Autodesk Inventor part; units mm, degrees
ref_plane "作業平面1" through (0, 0, 0) normal (0, 1, 0) x (-1, 0, 0)
ref_plane "YZ Plane" through (0, 0, 0) normal (1, 0, 0) x (0, 1, 0)
ref_plane "XY Plane" through (0, 0, 0) normal (0, 0, 1) x (1, 0, 0)
sketch "スケッチ1" plane through (0, 0, 0) normal (0, 0, 1) x (1, 0, 0)
  circle A0 centre (0, 0) radius 40
  circle A1 centre (0, 0) radius 2.5
  dimension "d0" = 80
  dimension "d1" = 5
extrude "押し出し1" add sketch "スケッチ1" along normal blind 3
sketch "スケッチ2" plane through (0, 0, 3) normal (0, 0, 1) x (1, 0, 0)
  circle A0 centre (0, 0) radius 8
  circle A1 centre (0, 0) radius 2.5
  circle A2 centre (0, 0) radius 35
  line L0 (3, 34.8712) -> (3, 7.4162)
  line L1 (-3, 7.4162) -> (-3, 34.8712)
  line L2 (-7.3654, 3.1227) -> (-26.779, 22.5363)
  line L3 (-22.5363, 26.779) -> (-3.1227, 7.3654)
  circle A3 centre (0, 0) radius 35
  circle A4 centre (0, 0) radius 8
  line L4 (-7.4162, -3) -> (-34.8712, -3)
  line L5 (-34.8712, 3) -> (-7.4162, 3)
  circle A5 centre (0, 0) radius 35
  circle A6 centre (0, 0) radius 8
  line L6 (-3.1227, -7.3654) -> (-22.5363, -26.779)
  line L7 (-26.779, -22.5363) -> (-7.3654, -3.1227)
  circle A7 centre (0, 0) radius 35
  circle A8 centre (0, 0) radius 8
  line L8 (3, -7.4162) -> (3, -34.8712)
  line L9 (-3, -34.8712) -> (-3, -7.4162)
  circle A9 centre (0, 0) radius 35
  circle A10 centre (0, 0) radius 8
  line L10 (7.3654, -3.1227) -> (26.779, -22.5363)
  line L11 (22.5363, -26.779) -> (3.1227, -7.3654)
  circle A11 centre (0, 0) radius 35
  circle A12 centre (0, 0) radius 8
  line L12 (7.4162, 3) -> (34.8712, 3)
  line L13 (34.8712, -3) -> (7.4162, -3)
  circle A13 centre (0, 0) radius 35
  circle A14 centre (0, 0) radius 8
  line L14 (3.1227, 7.3654) -> (22.5363, 26.779)
  line L15 (26.779, 22.5363) -> (7.3654, 3.1227)
  circle A15 centre (0, 0) radius 35
  circle A16 centre (0, 0) radius 8
  dimension "d4" = 16
  dimension "d5" = 70
  dimension "d6" = 3
  dimension "d7" = 6
  dimension "d10" = 360
extrude "押し出し2" cut sketch "スケッチ2" against normal blind 5 contours A0 L15 A2 L12 | L13 A2 L10 A0 | A0 L0 A2 L14 | L11 A2 L8 A0 | A0 L3 A2 L1 | L9 A2 L6 A0 | A0 L5 A2 L2 | L7 A2 L4 A0
sketch "スケッチ3" plane through (0, 0, 3) normal (0, 0, 1) x (1, 0, 0)
  circle A0 centre (0, 0) radius 2.5
  circle A1 centre (0, 0) radius 2.5
  circle A2 centre (0, 0) radius 6
  dimension "d14" = 12
extrude "押し出し3" add sketch "スケッチ3" along normal blind 8
ref_plane "作業平面1" through (0, 0, 0) normal (0, 1, 0) x (-1, 0, 0)
sketch "スケッチ4" plane through (0, 0, 0) normal (0, 1, 0) x (-1, 0, 0)
  circle A0 centre (0, 7) radius 1.25
  line L0 (40, 3) -> (-40, 3)
  point P0 (0, 0)
  dimension "d18" = 2.5
  dimension "d19" = 4
extrude "押し出し4" cut sketch "スケッチ4" along normal mid plane 15
sketch "スケッチ5" plane through (0, 0, 11) normal (0, 0, 1) x (1, 0, 0)
  circle A0 centre (0, 0) radius 2.8
  dimension "d22" = 5.6
extrude "押し出し5" cut sketch "スケッチ5" against normal blind 20
Source: CAD feature listing. Evaluate the final solid. Frame: model axes, mm. A direction names the side the tool comes from. Round coordinates to 2 decimals unless told otherwise and drop trailing zeros. Write each loop counter-clockwise with the first axis right and the second up, starting at its lowest first coordinate (ties: lowest second). Pieces come first, ordered by that corner, then holes. Notation, with made-up numbers: M -2,28.5 L 5,28.5 A24 ccw 5,51.5 Z; hole C -4.75,-39.5 d6. An arc over 180 degrees is marked long. Answer as a JSON object with one key per item and string values. Group by question number.
(1) Section query C-C on x = 31. Output: boundary loops of the cut face in (y, z).
(2) Mould query, pull axis Y, two halves, no side actions, for faces 1 (the flat face through (3, -1, 11)), 2 (the cylindrical face through (-32.28, 13.53, 1.52)). Classes: +Y half, -Y half, draft (parallel to the pull), parting line (faces both ways), or undercut.
(3) Reachability of faces 3 (the cylindrical face through (1.25, -4.23, 7.05)), 4 (the flat face through (16.936, -12.694, 1.521)) from +Z, -Z, +X, -X, +Y, -Y: full face, straight path, thin tool, end or side. Return the list, or none.
(4) Section query A-A on y = 0. Output: boundary loops of the cut face in (x, z).
(5) First-contact query: pin 1 (0.9 mm diameter, centred on x = 19.5, z = 1, fed in from -Y); pin 2 (1.5 mm diameter, centred on y = -24, z = 1.5, fed in from -X); pin 3 (5 mm diameter, centred on x = -30, y = 13, fed in from +Z). Flat tips, straight axial feed; report the tip coordinate or a pass-through.
(6) Section query D-D on z = 7. Output: boundary loops of the cut face in (x, y), then the cut area to 3 significant figures.
(7) Section query B-B on z = 1.25. State how many separate pieces and enclosed holes the cut face has, then the cut area to 3 significant figures.
(8) Ray query, line 1 (Y direction, x = 17, z = 2); line 2 (Z direction, x = 0, y = -5); line 3 (Y direction, x = 0, z = 4). Return the intervals inside material, ascending. Write a range as [from, to].
Computed values:
{
 "1": {"outline": "M -25.28,0 L -16.25,0 L -16.25,3 L -25.28,3 Z; M -3,0 L 3,0 L 3,3 L -3,3 Z; M 16.25,0 L 25.28,0 L 25.28,3 L 16.25,3 Z"},
 "2": {"face 1": "draft", "face 2": "undercut"},
 "3": {"face 3": "+Y, -Y", "face 4": "+Z, -Z"},
 "4": {"outline": "M -40,0 L -2.8,0 L -2.8,11 L -6,11 L -6,3 L -40,3 Z; M 2.8,0 L 40,0 L 40,3 L 6,3 L 6,11 L 2.8,11 Z"},
 "5": {"pin 1": "y = -35.17", "pin 2": "x = -32.55", "pin 3": "z = 3"},
 "6": {"outline": "M -1.25,-5.87 L -1.25,-2.51 A2.8 cw -1.25,2.51 L -1.25,5.87 A6 ccw Z; M 1.25,-5.87 A6 ccw 1.25,5.87 L 1.25,2.51 A2.8 cw 1.25,-2.51 Z", "area": "72.2 mm^2"},
 "7": {"separate pieces": "1", "enclosed holes": "9", "area": "2,660 mm^2"},
 "8": {"line 1": "[-36.21, -30.59], [-21.24, -12.76], [-3, 3], [12.76, 21.24], [30.59, 36.21]", "line 2": "[0, 5.75], [8.25, 11]", "line 3": "[-6, -2.8], [2.8, 6]"}
}
